```python
from build123d import *

# Parameters (mm, degrees)
SKETCH1_R               = 7.45
BOSS_EXTRUDE1_DEPTH     = 20
SKETCH2_R               = 3
CUT_EXTRUDE1_DEPTH      = 14
SKETCH3_R               = 2.5
CUT_EXTRUDE2_DEPTH      = 6
CUT_EXTRUDE3_REACH      = 24.605
CUT_EXTRUDE3_END_RADIUS = 7.45
SKETCH4_R               = 1
CUT_EXTRUDE4_REACH      = 24.605
CUT_EXTRUDE4_END_RADIUS = 7.45
SKETCH6_R               = 1


with BuildPart() as part:
    # Sketch1 → Boss-Extrude1 (new body)
    with BuildSketch(Plane(origin=(0, 0, 0), x_dir=(1, 0, 0), z_dir=(0, 1, 0))):
        with Locations(Location((0, 0, 0), (0, 0, 270))):
            Circle(SKETCH1_R)
    extrude(amount=BOSS_EXTRUDE1_DEPTH)

    # Sketch2 → Cut-Extrude1 (cut)
    with BuildSketch(Plane(origin=(0, 20, 0), x_dir=(1, 0, 0), z_dir=(0, 1, 0))):
        with Locations(Location((0, 0, 0), (0, 0, 270))):
            Circle(SKETCH2_R)
    extrude(amount=-CUT_EXTRUDE1_DEPTH, mode=Mode.SUBTRACT)

    # Sketch3 → Cut-Extrude2 (cut)
    with BuildSketch(Plane.XZ):
        with Locations(Location((0, 0, 0), (0, 0, 270))):
            Circle(SKETCH3_R)
    extrude(amount=-CUT_EXTRUDE2_DEPTH, mode=Mode.SUBTRACT)

    # Cut-Extrude3: up to this cylinder (the profile starts inside it)
    cut_extrude3_end = Plane(origin=(0, 17, 0), z_dir=(0, -1, 0)) * Cylinder(CUT_EXTRUDE3_END_RADIUS, 65.11, mode=Mode.PRIVATE)
    # Sketch4 → Cut-Extrude3 (cut, up to the surface)
    with BuildSketch(Plane(origin=(0, 0, 0), x_dir=(0, 0, -1), z_dir=(1, 0, 0)), mode=Mode.PRIVATE) as cut_extrude3_sk1:
        with Locations((0, 17)):
            Circle(SKETCH4_R)
    cut_extrude3_tool1 = extrude(cut_extrude3_sk1.sketch, amount=-CUT_EXTRUDE3_REACH, mode=Mode.PRIVATE) & cut_extrude3_end
    add(cut_extrude3_tool1.solids().sort_by_distance((0, 17, 0))[0], mode=Mode.SUBTRACT)

    # Cut-Extrude4: up to this cylinder (the profile starts inside it)
    cut_extrude4_end = Plane(origin=(0, 3, 0), z_dir=(0, -1, 0)) * Cylinder(CUT_EXTRUDE4_END_RADIUS, 65.11, mode=Mode.PRIVATE)
    # Sketch6 → Cut-Extrude4 (cut, up to the surface)
    with BuildSketch(Plane.XY, mode=Mode.PRIVATE) as cut_extrude4_sk1:
        with Locations((0, 3)):
            Circle(SKETCH6_R)
    cut_extrude4_tool1 = extrude(cut_extrude4_sk1.sketch, amount=-CUT_EXTRUDE4_REACH, mode=Mode.PRIVATE) & cut_extrude4_end
    add(cut_extrude4_tool1.solids().sort_by_distance((0, 3, 0))[0], mode=Mode.SUBTRACT)


solid = part.part
```
Can you work these out from the model? Positions are in its coordinate system, mm. A direction names the side the tool comes from. Give positions to 0.01 mm unless a question says otherwise; leave off trailing zeros. Order: outer loops, then holes, each group sorted by start corner. A loop starts at its lowest first (then second) coordinate and runs counter-clockwise, first axis right, second up. Notation, with made-up numbers: M -38,25 L -32,25 A17 cw -32,32 Z; hole C 45.5,-23.5 d6. An arc over 180 degrees is marked long. Write item = value, one per line. Start each with the question number.
Q1. We'd pull the mould along X, two halves only. Please class faces 1 (the flat face through (0.1, 20, 3.2)), 2 (the cylindrical face through (-2.853, 9.86, 6.882)), 3 (the cylindrical face through (0.9, 13.1, 2.86)): pulls with the +X half, pulls with the -X half, needs draft (parallel to the pull), parting line crosses it, or undercut.
Q2. Suppose I cut it at B-B (z = 0). Write out the boundary of the cut face in (x, y).
Q3. Suppose I cut it at C-C (y = 6.5). Write out the boundary of the cut face in (x, z), plus the area to 3 significant figures.
Q4. Suppose I cut it at D-D (z = 1.5). Write out the boundary of the cut face in (x, y).
Q5. Suppose I cut it at A-A (x = 0). Write out the boundary of the cut face in (y, z).
Q6. For faces 4 (the cylindrical face through (0.1, 3, 2.5)), 5 (the cylindrical face through (0, 4, -5)), 6 (the flat face through (2, 6, -2)), 7 (the cylindrical face through (-5, 16, 0)), which set-ups out of +Z, -Z, +X, -X, +Y, -Y let a thin tool reach every point of the face, with its end or its side?
Q7. I need wall thicknesses on probe 1 along X at (y, z) = (1.5, 0); probe 2 along X at (y, z) = (9, 0); probe 3 along Z at (x, y) = (-2.25, 14.5). Which ranges of each line are inside material? Lowest first, please. Write a range as [from, to].
Q8. Will these pins go through, and if not, where does the flat tip stop? pin 1 Ø6 at (x, y) = (4, 4.5) entering from -Z; pin 2 Ø3 at (y, z) = (16.5, -5.5) entering from +X; pin 3 Ø1.8 at (y, z) = (17, 0) entering from -X; pin 4 Ø5 at (x, z) = (-1.5, 0.5) entering from +Y.
Check result:
q1.face_1 = needs draft
q1.face_2 = parting line crosses it
q1.face_3 = undercut
q2.outline = M -7.45,0 L -2.5,0 L -2.5,6 L -3,6 L -3,16 L -7.45,16 Z; M -7.45,18 L -3,18 L -3,20 L -7.45,20 Z; M 2.5,0 L 7.45,0 L 7.45,20 L 3,20 L 3,6 L 2.5,6 Z
q3.outline = C 0,0 d14.9; hole C 0,0 d6
q3.area = 146 mm2
q4.outline = M -7.3,0 L -2,0 L -2,6 L -2.6,6 L -2.6,20 L -7.3,20 Z; M 2,0 L 7.3,0 L 7.3,20 L 2.6,20 L 2.6,6 L 2,6 Z
q5.outline = M 0,-7.45 L 2,-7.45 L 2,-2.5 L 0,-2.5 Z; M 0,2.5 L 6,2.5 L 6,3 L 20,3 L 20,7.45 L 0,7.45 Z; M 4,-7.45 L 20,-7.45 L 20,-3 L 6,-3 L 6,-2.5 L 4,-2.5 Z
q6.face_4 = +Y, -Y
q6.face_5 = -Z
q6.face_6 = +Y
q6.face_7 = -X
q7.probe_1 = [-7.45, -2.5], [2.5, 7.45]
q7.probe_2 = [-7.45, -3], [3, 7.45]
q7.probe_3 = [-7.1, -1.98], [1.98, 7.1]
q8.pin_1 = -7.38
q8.pin_2 = 6.29
q8.pin_3 = 2.86
q8.pin_4 = 20
